Design review of the part built by this model. Coordinates are the model's own, in mm. A direction names the side the tool comes from. Coordinates: 2 decimals unless noted, no trailing zeros. Loops run counter-clockwise (first coordinate to the right, second up) from the corner with the lowest first, then second, coordinate; pieces in that order, holes last. Notation, with made-up numbers: (-13.5, 22) -> (-7.5, 22) arc R37 ccw to (-7.5, 60) -> close; hole circle Ø10 at (-36, 13). An arc over 180 degrees is marked (long way). Use CSV: the item, a comma, the result in double quotes.
Autodesk Inventor part; units mm, degrees
ref_plane "YZ Plane" through (0, 0, 0) normal (1, 0, 0) x (0, 1, 0)
ref_plane "XZ Plane" through (0, 0, 0) normal (0, 1, 0) x (-1, 0, 0)
ref_plane "XY Plane" through (0, 0, 0) normal (0, 0, 1) x (1, 0, 0)
sketch "Boceto1" plane through (0, 0, 0) normal (0, 1, 0) x (-1, 0, 0)
  circle A0 centre (0, 0) radius 2.5
  circle A1 centre (0, 0) radius 4.75
  dimension "d0" = 5
  dimension "d1" = 9.5
extrude "Extrusión1" add sketch "Boceto1" along normal blind 2.75 contours A0 | A1
extrude "Extrusión2" add sketch "Boceto1" against normal blind 10 contours A0
thread "Rosca1"
fillet "Empalme1" radius 2.25 1 edges at (4.75, 2.75, 0)
sketch "Boceto2" plane through (0, 2.75, 0) normal (0, 1, 0) x (1, 0, 0)
  line L0 (0.7249, 1.5731) -> (1.7248, 0.1588)
  line L1 (1.7248, 0.1588) -> (0.9999, -1.4143)
  line L2 (0.9999, -1.4143) -> (-0.7249, -1.5731)
  line L3 (-0.7249, -1.5731) -> (-1.7248, -0.1588)
  line L4 (-1.7248, -0.1588) -> (-0.9999, 1.4143)
  line L5 (-0.9999, 1.4143) -> (0.7249, 1.5731)
  point P0 (0, 0)
  point P1 (0, 0)
  dimension "d9" = 3
extrude "Extrusión3" cut sketch "Boceto2" against normal blind 1.56
chamfer "Chaflán1" distance 0.5 angle 45 1 edges at (2.5, -10, 0)
properties part number "Tornillo allen cabeza boton M5"
Item 1: Machinability: for faces 4 (the face through (0.15, 1.981, 1.493)), 5 (the face through (0.54, -4.68, -2.44)), 6 (the face through (0, 2.75, -2)), which of the approach directions +Z, -Z, +X, -X, +Y, -Y give a long, thin tool a straight path to every point of the face, cutting with its end or side? Answer none if there is none.
Checked values:
face 4,"+Y"
face 5,"-Y"
face 6,"+Z, -Z, +X, -X, +Y"
Item 2: Draft analysis for pull direction Z (two halves, no side actions). For faces 1 (the face through (-2.192, 0.246, 4.214)), 2 (the face through (-2, 0, -2)), 3 (the face through (-1.367, 1.981, -0.617)), state which applies: pulls with the +Z half, pulls with the -Z half, needs draft (parallel to the pull), parting line crosses it, or undercut.
Checked values:
face 1,"parting line crosses it"
face 2,"needs draft"
face 3,"undercut"
Item 3: Add section A-A (y = 1.75). Give the boundary of the cut face in (x, z), then the cut area to 3 significant figures.
Checked values:
outline,"circle Ø8.74 at (0, 0); hole (-1.72, 0.16) -> (-1, -1.41) -> (0.72, -1.57) -> (1.72, -0.16) -> (1, 1.41) -> (-0.72, 1.57) -> close"
area,"52.2 mm^2"
Item 4: Clearance check with flat-ended pins moving along their axes: pin 1 (2 mm diameter, centred on y = -6.5, z = -0.5, fed in from -X); pin 2 (1.5 mm diameter, centred on x = -2.5, z = 3.5, fed in from -Y). State where each tip first meets the part, or that it passes through.
Checked values:
pin 1,"x = -2.5"
pin 2,"y = 0"
Item 5: Add section C-C (y = -2.5). Give the boundary of the cut face in (x, z).
Checked values:
outline,"circle Ø5 at (0, 0)"
Item 6: Add section B-B (x = 0). Give the boundary of the cut face in (y, z).
Checked values:
outline,"(-10, -2) -> (-9.5, -2.5) -> (0, -2.5) -> (0, -4.75) -> (0.5, -4.75) arc R2.25 ccw to (2.75, -2.5) -> (2.75, -1.51) -> (1.19, -1.51) -> (1.19, 1.51) -> (2.75, 1.51) -> (2.75, 2.5) arc R2.25 ccw to (0.5, 4.75) -> (0, 4.75) -> (0, 2.5) -> (-9.5, 2.5) -> (-10, 2) -> close"
Item 7: Add section D-D (z = 0). Give the boundary of the cut face in (x, y).
Checked values:
outline,"(-4.75, 0) -> (-2.5, 0) -> (-2.5, -9.5) -> (-2, -10) -> (2, -10) -> (2.5, -9.5) -> (2.5, 0) -> (4.75, 0) -> (4.75, 0.5) arc R2.25 ccw to (2.5, 2.75) -> (1.65, 2.75) -> (1.65, 1.19) -> (-1.65, 1.19) -> (-1.65, 2.75) -> (-2.5, 2.75) arc R2.25 ccw to (-4.75, 0.5) -> close"
Item 8: To check wall thickness, follow line 1 along X through (y, z) = (-4.75, -1.5); line 2 along X through (y, z) = (1.5, -1); line 3 along Z through (x, y) = (0.75, -8.25). State the ranges of each line that lie inside material, in increasing order.
Checked values:
line 1,"-2 to 2"
line 2,"-4.4 to -1.19, 1.13 to 4.4"
line 3,"-2.38 to 2.38"
